Geometry: see drawing. Coordinates: mm, zero at the bounding-box minimum. A direction names the side the tool comes from. Round coordinates to 2 decimals unless told otherwise and drop trailing zeros. Loops run counter-clockwise (first coordinate to the right, second up) from the corner with the lowest first, then second, coordinate; pieces in that order, holes last. Notation, with made-up numbers: (85.25, 44) - (104.25, 44) arc R27 ccw to (104.25, 68) - close; hole circle Ø8 at (8.25, -32). An arc over 180 degrees is marked (long way). Write item = value, one per line. Start each with the question number.
Item 1: Draft query along X for the marked faces 1, 2 and 3. Return one class per face: pulls with the +X half, pulls with the -X half, needs draft (parallel to the pull), parting line crosses it, or undercut.
Item 2: Section C-C (y = 3.25). Return loops of the section in (x, z), plus the area to 3 significant figures.
Item 3: Section B-B (x = 14). Return loops of the section in (y, z), plus the area to 3 significant figures.
Item 4: Section D-D (z = 8). Return loops of the section in (x, y), plus the area to 3 significant figures.
Item 5: Line query: line 1 (Y direction, x = 4.5, z = 9.75); line 2 (X direction, y = 19, z = 9.5); line 3 (Y direction, x = 12, z = 5.5). Output: solid intervals per line, ascending. Write a range as from..to.
Item 6: Access query for the marked faces 4 and 5. Directions: +Z, -Z, +X, -X, +Y, -Y. A direction counts if a zero-diameter tool reaches every point of the face in a straight line with its end or side. Return the directions, or none.
Item 7: First-contact query: pin 1 (6 mm diameter, centred on x = 14, z = 8, fed in from +Y). Flat tip, straight axial feed; report the tip coordinate or a pass-through.
Item 8: Section A-A (x = 22). Return loops of the section in (y, z).
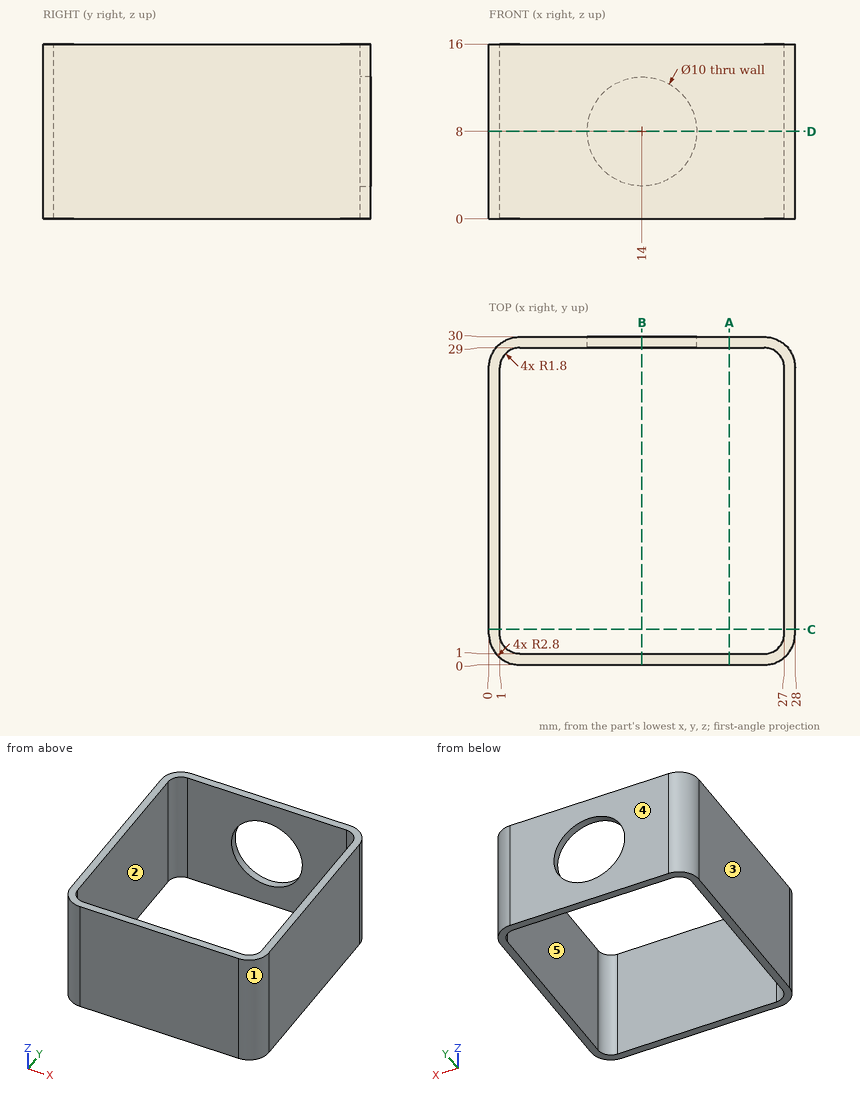
Taken from the geometry:
q1.face_1 = pulls with the +X half
q1.face_2 = undercut
q1.face_3 = pulls with the -X half
q2.outline = (0, 0) - (1, 0) - (1, 16) - (0, 16) - close; (27, 0) - (28, 0) - (28, 16) - (27, 16) - close
q2.area = 32.0 mm^2
q3.outline = (0, 0) - (1, 0) - (1, 16) - (0, 16) - close; (29, 0) - (30, 0) - (30, 3) - (29, 3) - close; (29, 13) - (30, 13) - (30, 16) - (29, 16) - close
q3.area = 22.0 mm^2
q4.outline = (0, 2.8) arc R2.8 ccw to (2.8, 0) - (25.2, 0) arc R2.8 ccw to (28, 2.8) - (28, 27.2) arc R2.8 ccw to (25.2, 30) - (19, 30) - (19, 29) - (25.2, 29) arc R1.8 cw to (27, 27.2) - (27, 2.8) arc R1.8 cw to (25.2, 1) - (2.8, 1) arc R1.8 cw to (1, 2.8) - (1, 27.2) arc R1.8 cw to (2.8, 29) - (9, 29) - (9, 30) - (2.8, 30) arc R2.8 ccw to (0, 27.2) - close
q4.area = 98.1 mm^2
q5.line_1 = 0..1, 29..30
q5.line_2 = 0..1, 27..28
q5.line_3 = 0..1
q6.face_4 = +Z, -Z, +X, -X, +Y
q6.face_5 = +Z, -Z
q7.pin_1 = 1
q8.outline = (0, 0) - (1, 0) - (1, 16) - (0, 16) - close; (29, 0) - (30, 0) - (30, 16) - (29, 16) - close
